Here's the drawing with two shaded views (mm, measured from the low corner). I have some questions. Round coordinates to 2 decimals unless told otherwise and drop trailing zeros. Order: outer loops, then holes, each group sorted by start corner. A loop starts at its lowest first (then second) coordinate and runs counter-clockwise, first axis right, second up. Notation, with made-up numbers: (35.25, 78.5) - (47.25, 78.5) arc R20 ccw to (47.25, 82.5) - close; hole circle Ø11 at (-28.5, -22). An arc over 180 degrees is marked (long way). Return JSON: item names as keys, results as strings. Group by question number.
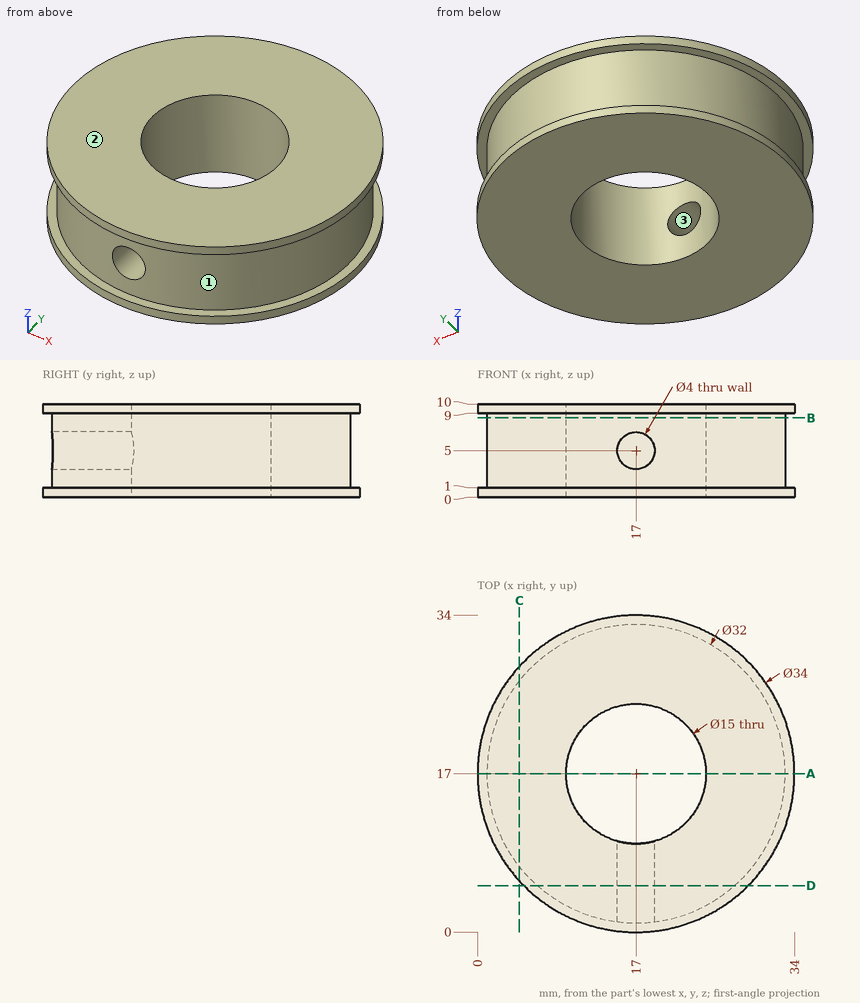
1) We'd pull the mould along X, two halves only. Please class the marked faces 1, 2 and 3: +X half, -X half, draft (parallel to the pull), parting line (faces both ways), or undercut.
2) I want a section at C-C, the plane x = 4.5. List the corners of the cut face in (y, z) for me.
3) I want a section at B-B, the plane z = 8.5. List the corners of the cut face in (x, y) for me, plus the area to 3 significant figures.
4) If I drill on line 1 along Z through (x, y) = (30.5, 8); line 2 along Z through (x, y) = (17, 7.25); line 3 along Y through (x, z) = (17, 8.5), over which ranges is the centre line in solid material (lowest first)? Write a range as from..to.
5) Will these pins go through, and if not, where does the flat tip stop? pin 1 (2 mm diameter, centred on y = 19.5, z = 8.5, fed in from -X); pin 2 (2 mm diameter, centred on y = 11, z = 5, fed in from +X); pin 3 (5 mm diameter, centred on y = 15, z = 4.5, fed in from +X).
6) I want a section at A-A, the plane y = 17. List the corners of the cut face in (x, z) for me, plus the area to 3 significant figures.
7) I want a section at D-D, the plane y = 5. List the corners of the cut face in (x, z) for me, plus the area to 3 significant figures.
Outcome:
{
 "1": {"face 1": "parting line", "face 2": "draft", "face 3": "undercut"},
 "2": {"outline": "(5.48, 0) - (28.52, 0) - (28.52, 1) - (26.99, 1) - (26.99, 9) - (28.52, 9) - (28.52, 10) - (5.48, 10) - (5.48, 9) - (7.01, 9) - (7.01, 1) - (5.48, 1) - close"},
 "3": {"outline": "circle Ø32 at (17, 17); hole circle Ø15 at (17, 17)", "area": "628 mm^2"},
 "4": {"line 1": "0..1, 9..10", "line 2": "0..3, 7..10", "line 3": "1..9.5, 24.5..33"},
 "5": {"pin 1": "x = 0.08", "pin 2": "x = 32.2", "pin 3": "x = 33"},
 "6": {"outline": "(0, 0) - (9.5, 0) - (9.5, 10) - (0, 10) - (0, 9) - (1, 9) - (1, 1) - (0, 1) - close; (24.5, 0) - (34, 0) - (34, 1) - (33, 1) - (33, 9) - (34, 9) - (34, 10) - (24.5, 10) - close", "area": "174 mm^2"},
 "7": {"outline": "(4.96, 0) - (29.04, 0) - (29.04, 1) - (27.58, 1) - (27.58, 9) - (29.04, 9) - (29.04, 10) - (4.96, 10) - (4.96, 9) - (6.42, 9) - (6.42, 1) - (4.96, 1) - close; hole circle Ø4 at (17, 5)", "area": "205 mm^2"}
}
